from build123d import *

# Parameters (mm, degrees)
EXTRUDE_1_DEPTH     = 3
CUT_EXTRUDE_2_DEPTH = 62.238264182
SKETCH_7_R          = 1.6
SKETCH_7_R_2        = 27.5
CUT_EXTRUDE_3_DEPTH = 58.283549122
SKETCH_2_R          = 1.6
CUT_EXTRUDE_4_DEPTH = 58.283549122
SKETCH_8_W          = 61
SKETCH_8_H          = 7
CUT_EXTRUDE_5_DEPTH = 58.283549122
EXTRUDE_START       = 3
EXTRUDE_2_DEPTH     = 3


with BuildPart() as part:
    # 草图1 → 凸台-拉伸1 (new body)
    with BuildSketch(Plane.XY):
        with BuildLine():
            Line((-27.5, 43.25), (27.5, 43.25))
            ThreePointArc((27.5, 43.25), (28.207106781, 42.957106781), (28.5, 42.25))
            Line((28.5, 42.25), (28.5, 36.65))
            ThreePointArc((28.5, 36.65), (30.887079733, 30.887079733), (36.65, 28.5))
            Line((36.65, 28.5), (42.25, 28.5))
            ThreePointArc((42.25, 28.5), (42.957106781, 28.207106781), (43.25, 27.5))
            Line((43.25, 27.5), (43.25, -27.5))
            ThreePointArc((43.25, -27.5), (42.957106781, -28.207106781), (42.25, -28.5))
            Line((42.25, -28.5), (36.65, -28.5))
            ThreePointArc((36.65, -28.5), (30.887079733, -30.887079733), (28.5, -36.65))
            Line((28.5, -36.65), (28.5, -42.25))
            ThreePointArc((28.5, -42.25), (28.207106781, -42.957106781), (27.5, -43.25))
            Line((27.5, -43.25), (-27.5, -43.25))
            ThreePointArc((-27.5, -43.25), (-28.207106781, -42.957106781), (-28.5, -42.25))
            Line((-28.5, -42.25), (-28.5, -36.65))
            ThreePointArc((-28.5, -36.65), (-30.887079733, -30.887079733), (-36.65, -28.5))
            Line((-36.65, -28.5), (-42.25, -28.5))
            ThreePointArc((-42.25, -28.5), (-42.957106781, -28.207106781), (-43.25, -27.5))
            Line((-43.25, -27.5), (-43.25, 27.5))
            ThreePointArc((-43.25, 27.5), (-42.957106781, 28.207106781), (-42.25, 28.5))
            Line((-42.25, 28.5), (-36.65, 28.5))
            ThreePointArc((-36.65, 28.5), (-30.887079733, 30.887079733), (-28.5, 36.65))
            Line((-28.5, 36.65), (-28.5, 42.25))
            ThreePointArc((-28.5, 42.25), (-28.207106781, 42.957106781), (-27.5, 43.25))
        make_face()
    extrude(amount=EXTRUDE_1_DEPTH)

    # 草图6 → 切除-拉伸2 (cut, through all)
    with BuildSketch(Plane.XY.offset(3)):
        with BuildLine():
            Line((-28.5, 42.25), (-28.5, 36.65))
            ThreePointArc((-28.5, 36.65), (-30.887079733, 30.887079733), (-36.65, 28.5))
            Line((-36.65, 28.5), (-42.25, 28.5))
            ThreePointArc((-42.25, 28.5), (-42.957106781, 28.207106781), (-43.25, 27.5))
            Line((-43.25, 27.5), (-43.25, -27.5))
            ThreePointArc((-43.25, -27.5), (-42.957106781, -28.207106781), (-42.25, -28.5))
            Line((-42.25, -28.5), (-36.65, -28.5))
            ThreePointArc((-36.65, -28.5), (-30.887079733, -30.887079733), (-28.5, -36.65))
            Line((-28.5, -36.65), (-28.5, -42.25))
            ThreePointArc((-28.5, -42.25), (-28.207106781, -42.957106781), (-27.5, -43.25))
            Line((-27.5, -43.25), (27.5, -43.25))
            ThreePointArc((27.5, -43.25), (28.207106781, -42.957106781), (28.5, -42.25))
            Line((28.5, -42.25), (28.5, -36.65))
            ThreePointArc((28.5, -36.65), (30.887079733, -30.887079733), (36.65, -28.5))
            Line((36.65, -28.5), (42.25, -28.5))
            ThreePointArc((42.25, -28.5), (42.957106781, -28.207106781), (43.25, -27.5))
            Line((43.25, -27.5), (43.25, 27.5))
            ThreePointArc((43.25, 27.5), (42.957106781, 28.207106781), (42.25, 28.5))
            Line((42.25, 28.5), (36.65, 28.5))
            ThreePointArc((36.65, 28.5), (30.887079733, 30.887079733), (28.5, 36.65))
            Line((28.5, 36.65), (28.5, 42.25))
            ThreePointArc((28.5, 42.25), (28.207106781, 42.957106781), (27.5, 43.25))
            Line((27.5, 43.25), (-27.5, 43.25))
            ThreePointArc((-27.5, 43.25), (-28.207106781, 42.957106781), (-28.5, 42.25))
        make_face()
        with BuildLine():
            Line((-25.7, 40.45), (-25.7, 36.65))
            ThreePointArc((-25.7, 36.65), (-28.907180746, 28.907180746), (-36.65, 25.7))
            Line((-36.65, 25.7), (-40.45, 25.7))
            Line((-40.45, 25.7), (-40.45, -25.7))
            Line((-40.45, -25.7), (-36.65, -25.7))
            ThreePointArc((-36.65, -25.7), (-28.907180746, -28.907180746), (-25.7, -36.65))
            Line((-25.7, -36.65), (-25.7, -40.45))
            Line((-25.7, -40.45), (25.7, -40.45))
            Line((25.7, -40.45), (25.7, -36.65))
            ThreePointArc((25.7, -36.65), (28.907180746, -28.907180746), (36.65, -25.7))
            Line((36.65, -25.7), (40.45, -25.7))
            Line((40.45, -25.7), (40.45, 25.7))
            Line((40.45, 25.7), (36.65, 25.7))
            ThreePointArc((36.65, 25.7), (28.907180746, 28.907180746), (25.7, 36.65))
            Line((25.7, 36.65), (25.7, 40.45))
            Line((25.7, 40.45), (-25.7, 40.45))
        make_face(mode=Mode.SUBTRACT)
    extrude(amount=-CUT_EXTRUDE_2_DEPTH, mode=Mode.SUBTRACT)

    # 草图7 → 切除-拉伸3 (cut, through all)
    with BuildSketch(Plane.XY.offset(3)):
        with Locations((-25, 25)):
            Circle(SKETCH_7_R)
        with Locations((25, 25)):
            Circle(SKETCH_7_R)
        with Locations((25, -25)):
            Circle(SKETCH_7_R)
        with Locations((-25, -25)):
            Circle(SKETCH_7_R)
        Circle(SKETCH_7_R_2)
    extrude(amount=-CUT_EXTRUDE_3_DEPTH, mode=Mode.SUBTRACT)

    # 草图2 → 切除-拉伸4 (cut, through all)
    with BuildSketch(Plane.XY.offset(3)):
        with Locations((-33.80515662, 21.19484338)):
            Circle(SKETCH_2_R)
        with Locations((21.19484338, 33.80515662)):
            Circle(SKETCH_2_R)
        with Locations((33.80515662, -21.19484338)):
            Circle(SKETCH_2_R)
        with Locations((-21.19484338, -33.80515662)):
            Circle(SKETCH_2_R)
    extrude(amount=-CUT_EXTRUDE_4_DEPTH, mode=Mode.SUBTRACT)

    # 草图8 → 切除-拉伸5 (cut, through all)
    with BuildSketch(Plane.XY.offset(3)):
        Rectangle(SKETCH_8_W, SKETCH_8_H)
    extrude(amount=-CUT_EXTRUDE_5_DEPTH, mode=Mode.SUBTRACT)

    # 草图9 → 凸台-拉伸2 (add)
    with BuildSketch(Plane.XY.offset(3).offset(EXTRUDE_START)):
        with BuildLine():
            Line((-34.5, -7.5), (-30.594117082, -7.5))
            ThreePointArc((-30.594117082, -7.5), (0, -31.5), (30.594117082, -7.5))
            Line((30.594117082, -7.5), (34.5, -7.5))
            Line((34.5, -7.5), (34.5, 7.5))
            Line((34.5, 7.5), (30.594117082, 7.5))
            ThreePointArc((30.594117082, 7.5), (0, 31.5), (-30.594117082, 7.5))
            Line((-30.594117082, 7.5), (-34.5, 7.5))
            Line((-34.5, 7.5), (-34.5, -7.5))
        make_face()
        with BuildLine():
            Line((-30.5, -3.5), (-27.276363394, -3.5))
            ThreePointArc((-27.276363394, -3.5), (0, -27.5), (27.276363394, -3.5))
            Line((27.276363394, -3.5), (30.5, -3.5))
            Line((30.5, -3.5), (30.5, 3.5))
            Line((30.5, 3.5), (27.276363394, 3.5))
            ThreePointArc((27.276363394, 3.5), (0, 27.5), (-27.276363394, 3.5))
            Line((-27.276363394, 3.5), (-30.5, 3.5))
            Line((-30.5, 3.5), (-30.5, -3.5))
        make_face(mode=Mode.SUBTRACT)
    extrude(amount=-EXTRUDE_2_DEPTH)


solid = part.part
Here's how the part is built. I have some questions about the finished solid (model axes, mm). A direction names the side the tool comes from. Give positions to 0.01 mm unless a question says otherwise; leave off trailing zeros. Loops run counter-clockwise (first coordinate to the right, second up) from the corner with the lowest first, then second, coordinate; pieces in that order, holes last. Notation, with made-up numbers: (7, 41.5) -> (32, 41.5) arc R34 ccw to (32, 73.5) -> close; hole circle Ø11 at (83, 77.25). An arc over 180 degrees is marked (long way). Answer as a JSON object with one key per item and string values. Group by question number.
Item 1: Will these pins go through, and if not, where does the flat tip stop? pin 1 (2.5 mm diameter, centred on y = 38.5, z = 1, fed in from -X); pin 2 (1.5 mm diameter, centred on x = -32.5, z = 5, fed in from +Y); pin 3 (2.5 mm diameter, centred on x = -38, z = 1.5, fed in from -Y).
Item 2: Imagine slicing it at A-A on z = 4.7. Write out the boundary of the cut face in (x, y).
Item 3: Imagine slicing it at D-D on x = -5. Write out the boundary of the cut face in (y, z), then the cut area to 3 significant figures.
Item 4: Imagine slicing it at B-B on x = -29. Write out the boundary of the cut face in (y, z), then the cut area to 3 significant figures.
Item 5: On a 3-axis mill with a long thin cutter (end or side, diameter ignored), from which of +Z, -Z, +X, -X, +Y, -Y can I reach the whole of each face in a straight line? I mean faces 1 (the flat face through (-34.5, 0, 5)), 2 (the flat face through (39, -25.7, 2)), 3 (the cylindrical face through (0.587, 31.495, 4.521)), 4 (the flat face through (33, -7.5, 5)). Say none if no direction works.
Item 6: Thinking about a two-plate mould opening in X: for faces 5 (the flat face through (-29, -3.5, 3)), 6 (the cylindrical face through (-28.993, -28.823, 1.521)), 7 (the flat face through (-33, 7.5, 5)), which applies, pulls with the +X half, pulls with the -X half, needs draft (parallel to the pull), parting line crosses it, or undercut?
Item 7: I need wall thicknesses on L1, parallel to Y at x = -0.5, z = 0.7; L2, parallel to Y at x = 25, z = 1.1; L3, parallel to X at y = 20.5, z = 1.05. Which ranges of each line are inside material? Lowest first, please.
Item 8: Imagine slicing it at C-C on x = -17. Write out the boundary of the cut face in (y, z), then the cut area to 3 significant figures.
Answer list:
{
 "1": {"pin 1": "stops at x = -25.7", "pin 2": "stops at y = 7.5", "pin 3": "stops at y = -25.7"},
 "2": {"outline": "(-34.5, -7.5) -> (-30.59, -7.5) arc R31.5 ccw to (30.59, -7.5) -> (34.5, -7.5) -> (34.5, 7.5) -> (30.59, 7.5) arc R31.5 ccw to (-30.59, 7.5) -> (-34.5, 7.5) -> close; hole (-30.5, -3.5) -> (-27.28, -3.5) arc R27.5 ccw to (27.28, -3.5) -> (30.5, -3.5) -> (30.5, 3.5) -> (27.28, 3.5) arc R27.5 ccw to (-27.28, 3.5) -> (-30.5, 3.5) -> close"},
 "3": {"outline": "(-40.45, 0) -> (-27.04, 0) -> (-27.04, 6) -> (-31.1, 6) -> (-31.1, 3) -> (-40.45, 3) -> close; (27.04, 0) -> (40.45, 0) -> (40.45, 3) -> (31.1, 3) -> (31.1, 6) -> (27.04, 6) -> close", "area": "105 mm2"},
 "4": {"outline": "(-28.82, 0) -> (-3.5, 0) -> (-3.5, 6) -> (-12.3, 6) -> (-12.3, 3) -> (-28.82, 3) -> close; (3.5, 0) -> (28.82, 0) -> (28.82, 3) -> (12.3, 3) -> (12.3, 6) -> (3.5, 6) -> close", "area": "205 mm2"},
 "5": {"face 1": "+Z, -X, +Y, -Y", "face 2": "+Z, -Z, +X, -Y", "face 3": "+Z, +Y", "face 4": "+Z, +X, -Y"},
 "6": {"face 5": "undercut", "face 6": "pulls with the -X half", "face 7": "needs draft"},
 "7": {"L1": "y = -40.45 to -27.5, 27.5 to 40.45", "L2": "y = -40.45 to -26.6, -23.4 to -11.46, 11.46 to 23.4, 26.6 to 40.45", "L3": "x = -40.45 to -35.25, -32.36 to -18.33, 18.33 to 40.45"},
 "8": {"outline": "(-40.45, 0) -> (-21.62, 0) -> (-21.62, 6) -> (-26.52, 6) -> (-26.52, 3) -> (-40.45, 3) -> close; (21.62, 0) -> (40.45, 0) -> (40.45, 3) -> (26.52, 3) -> (26.52, 6) -> (21.62, 6) -> close", "area": "142 mm2"}
}
